from build123d import *

# Parameters (mm, degrees)
F0_W     = 190
F0_H     = 190
F0_R     = 3.413695
F0_R_2   = 3.4135
F0_R_3   = 49.746444
F1_DEPTH = 3.2


with BuildPart() as f1:
    # F0 (on Top) → F1 (new body)
    with BuildSketch(Plane.XY):
        Rectangle(F0_W, F0_H)
        with Locations((-75, -75)):
            Circle(F0_R, mode=Mode.SUBTRACT)
        with Locations((75, -75)):
            Circle(F0_R_2, mode=Mode.SUBTRACT)
        with Locations((-75, 75)):
            Circle(F0_R_2, mode=Mode.SUBTRACT)
        Circle(F0_R_3, mode=Mode.SUBTRACT)
        with Locations((75, 75)):
            Circle(F0_R_2, mode=Mode.SUBTRACT)
        Circle(F0_R_3)
    extrude(amount=F1_DEPTH)


solid = f1.part
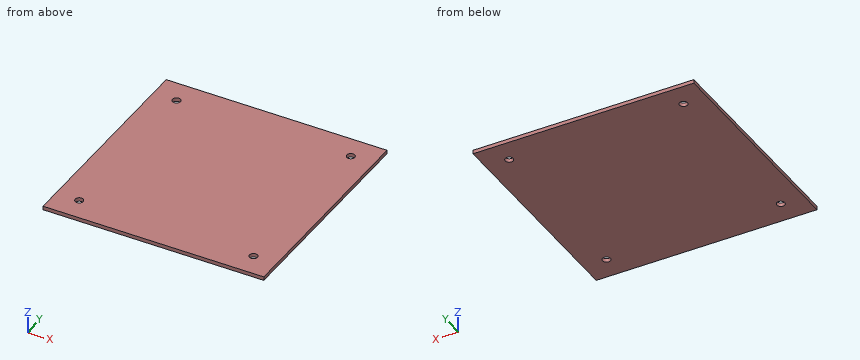
CAD build for the part. Positions are in the model's coordinates, mm. Round coordinates to 2 decimals unless told otherwise and drop trailing zeros. Order: outer loops, then holes, each group sorted by start corner. A loop starts at its lowest first (then second) coordinate and runs counter-clockwise, first axis right, second up. Notation, with made-up numbers: M 86.5,44 L 106.5,44 A23 ccw 106.5,64 Z; hole C 4,27 d3. An arc over 180 degrees is marked long. Use one line per item in the form item = value.
Q1. Probe L1, parallel to Y at x = -75, z = 0.9. List the from-to ranges inside material, lowest first.
Recorded:
L1 = -95 to -78.41, -71.59 to 71.59, 78.41 to 95
Q2. Saw through at A-A on y = 75. Give the cut face in (x, z).
Recorded:
outline = M -95,0 L -78.41,0 L -78.41,3.2 L -95,3.2 Z; M -71.59,0 L 71.59,0 L 71.59,3.2 L -71.59,3.2 Z; M 78.41,0 L 95,0 L 95,3.2 L 78.41,3.2 Z
Q3. Flat gauge pin, fed straight in: P1, Ø5, axis at x = 49.5, y = 40.5, coming from the -Z side. Where does the tip first touch, or does it go through?
Recorded:
P1 = 0
